from build123d import *

# Parameters (mm, degrees)
F1_DEPTH  = 10
F3_DEPTH  = 25.0000003725
F4_DEPTH  = 15
F5_R      = 13.75
F6_DEPTH  = 11.5
F7_DEPTH  = 7.5
F8_W      = 3
F8_H      = 12.169879545
F9_DEPTH  = 7
F10_W     = 3
F10_H     = 7.9815720619
F11_DEPTH = 4
F12_R     = 5
F13_R     = 5


# Not quite as in the source:
# - a feature names something its author has since deleted; it is built from what else it names


with BuildPart() as f1:
    # F0 (on Top) → F1 (new body)
    with BuildSketch(Plane.XY):
        with BuildLine():
            ThreePointArc((50, 15), (39.7487373415, 39.7487373415), (15, 50))
            Line((15, 50), (-15, 50))
            ThreePointArc((-15, 50), (-39.7487373415, 39.7487373415), (-50, 15))
            Line((-50, 15), (-50, -30))
            ThreePointArc((-50, -30), (-44.1421356237, -44.1421356237), (-30, -50))
            Line((-30, -50), (17.3621465266, -50))
            ThreePointArc((17.3621465266, -50), (19.1299134795, -49.267766953), (19.8621465266, -47.5))
            Line((19.8621465266, -47.5), (19.8621465266, -37.5))
            ThreePointArc((19.8621465266, -37.5), (19.1299134795, -35.732233047), (17.3621465266, -35))
            Line((17.3621465266, -35), (-30, -35))
            ThreePointArc((-30, -35), (-33.5355339059, -33.5355339059), (-35, -30))
            Line((-35, -30), (-35, 15))
            ThreePointArc((-35, 15), (-29.1421356237, 29.1421356237), (-15, 35))
            Line((-15, 35), (15, 35))
            ThreePointArc((15, 35), (29.1421356237, 29.1421356237), (35, 15))
            Line((35, 15), (35, -35))
            Line((35, -35), (35, -50))
            Line((35, -50), (50, -50))
            Line((50, -50), (50, 15))
        make_face()
    extrude(amount=F1_DEPTH)

    # F2 (on face) → F3 (cut)
    with BuildSketch(Plane.YZ.offset(50)):
        with BuildLine():
            ThreePointArc((-34.4148690401, 0), (-41.4859368519, 2.9289321881), (-44.4148690401, 10))
            Line((-44.4148690401, 10), (-50, 10))
            Line((-50, 10), (-50, 0))
            Line((-50, 0), (-34.4148690401, 0))
        make_face()
    extrude(amount=-F3_DEPTH, mode=Mode.SUBTRACT)

    # F2 (on face) → F4 (join)
    with BuildSketch(Plane.YZ.offset(50)):
        with BuildLine():
            Line((-10.5677563486, 86.0143546169), (-43.5051570601, 14.1673329256))
            ThreePointArc((-43.5051570601, 14.1673329256), (-44.1847943264, 12.1327353094), (-44.4148690401, 10))
            Line((-44.4148690401, 10), (-24.9867949218, 10))
            ThreePointArc((-24.9867949218, 10), (-29.1950209325, 12.299845589), (-29.5319389318, 17.0836664628))
            Line((-29.5319389318, 17.0836664628), (-0.1259929755, 81.2274541128))
            Line((-0.1259929755, 81.2274541128), (-10.5677563486, 86.0143546169))
        make_face()
    extrude(amount=-F4_DEPTH)

    # F5 (on face) → F6 (join)
    with BuildSketch(Plane(origin=(0, -41.3166681437, 18.9411282845), x_dir=(1, 0, 0), z_dir=(0, -0.909028802, 0.4167332926))):
        with BuildLine():
            ThreePointArc((-0.5725613731, 57.6122225326), (-5.3096309812, 69.0485202264), (-16.7459286749, 73.7855898345))
            ThreePointArc((-16.7459286749, 73.7855898345), (-32.9192959768, 57.6122225326), (-16.7459286749, 41.4388552308))
            ThreePointArc((-16.7459286749, 41.4388552308), (-5.3096309812, 46.1759248389), (-0.5725613731, 57.6122225326))
        make_face()
        with Locations((-16.7459286749, 57.6122225326)):
            Circle(F5_R, mode=Mode.SUBTRACT)
        with Locations((-16.7459286749, 57.6122225326)):
            Circle(F5_R)
        with BuildLine():
            Line((35, 41.4388552308), (35, 73.7855898345))
            Line((35, 73.7855898345), (-16.7459286749, 73.7855898345))
            ThreePointArc((-16.7459286749, 73.7855898345), (-5.3096309812, 69.0485202264), (-0.5725613731, 57.6122225326))
            ThreePointArc((-0.5725613731, 57.6122225326), (-5.3096309812, 46.1759248389), (-16.7459286749, 41.4388552308))
            Line((-16.7459286749, 41.4388552308), (35, 41.4388552308))
        make_face()
    extrude(amount=-F6_DEPTH)

    # F5 (on face) → F7 (cut)
    with BuildSketch(Plane(origin=(0, -41.3166681437, 18.9411282845), x_dir=(1, 0, 0), z_dir=(0, -0.909028802, 0.4167332926))):
        with Locations((-16.7459286749, 57.6122225326)):
            Circle(F5_R)
    extrude(amount=-F7_DEPTH, mode=Mode.SUBTRACT)

    # F8 (on face) → F9 (cut)
    with BuildSketch(Plane(origin=(0, -41.3166681437, 18.9411282845), x_dir=(1, 0, 0), z_dir=(0, -0.909028802, 0.4167332926))):
        with BuildLine():
            Line((2.0040713251, 56.1122225326), (2.0040713251, 59.1122225326))
            Line((2.0040713251, 59.1122225326), (2.0040713251, 61.1122225326))
            Line((2.0040713251, 61.1122225326), (-3.448842528, 61.1122225326))
            ThreePointArc((-3.448842528, 61.1122225326), (-3.109627224, 59.376813913), (-2.9959286749, 57.6122225326))
            ThreePointArc((-2.9959286749, 57.6122225326), (-3.109627224, 55.8476311523), (-3.448842528, 54.1122225326))
            Line((-3.448842528, 54.1122225326), (2.0040713251, 54.1122225326))
            Line((2.0040713251, 54.1122225326), (2.0040713251, 56.1122225326))
        make_face()
        with BuildLine():
            Line((36, 59.1122225326), (2.0040713251, 59.1122225326))
            Line((2.0040713251, 59.1122225326), (2.0040713251, 56.1122225326))
            Line((2.0040713251, 56.1122225326), (36, 56.1122225326))
            ThreePointArc((36, 56.1122225326), (39.5355339059, 54.6477564386), (41, 51.1122225326))
            Line((41, 51.1122225326), (41, -5.251533668))
            Line((41, -5.251533668), (44, -5.251533668))
            Line((44, -5.251533668), (44, 51.1122225326))
            ThreePointArc((44, 51.1122225326), (41.6568542495, 56.7690767821), (36, 59.1122225326))
        make_face()
        with Locations((42.5, -11.3364734405)):
            Rectangle(F8_W, F8_H)
    extrude(amount=-F9_DEPTH, mode=Mode.SUBTRACT)

    # F10 (on face) → F11 (cut)
    with BuildSketch(Plane(origin=(0, 0, 0), x_dir=(1, 0, 0), z_dir=(0, 0, -1))):
        with Locations((42.5, 38.4056550711)):
            Rectangle(F10_W, F10_H)
        with BuildLine():
            Line((44, 34.4148690401), (41, 34.4148690401))
            Line((41, 34.4148690401), (41, -38.4307490277))
            ThreePointArc((41, -38.4307490277), (42.5667640895, -36.5655632349), (44, -34.5959179423))
            Line((44, -34.5959179423), (44, 34.4148690401))
        make_face()
    extrude(amount=-F11_DEPTH, mode=Mode.SUBTRACT)

    # F12
    f12_edges = [f1.edges().sort_by_distance(p)[0] for p in [
        (42.5, -40.465722, 4),
    ]]
    fillet(f12_edges, radius=F12_R)

    # F13
    f13_edges = [f1.edges().sort_by_distance(p)[0] for p in [
        (50, -5.346875, 83.620904),
    ]]
    fillet(f13_edges, radius=F13_R)


solid = f1.part
Verification items for the finished model (mm, model axes). A direction names the side the tool comes from. Give positions to 0.01 mm unless a question says otherwise; leave off trailing zeros. Loops run counter-clockwise (first coordinate to the right, second up) from the corner with the lowest first, then second, coordinate; pieces in that order, holes last.
1) Depth check by flat-ended pin: pin 1 Ø0.9 at (x, y) = (42.5, -7.5) entering from -Z; pin 2 Ø10 at (y, z) = (-22, 41) entering from -X; pin 3 Ø2.5 at (y, z) = (-15, 66.5) entering from -X; pin 4 Ø5 at (x, y) = (37.5, 25) entering from -Z. Enter the tip coordinate at first touch or a pass-through.
2) Thickness scan on line 1 along X through (y, z) = (-41.5, 12.5); line 2 along Z through (x, y) = (39.5, 24); line 3 along Z through (x, y) = (43, -28). Record the ranges inside material, lowest first.
3) Draft check along Y on faces 6 (the flat face through (-16.94, -10.41, 68.36)), 7 (the flat face through (0, 50, 5)), 8 (the cylindrical face through (42.52, -36.84, 6.24)). Enter one of: pulls with the +Y half, pulls with the -Y half, needs draft (parallel to the pull), parting line crosses it, or undercut.
4) Sectioned sample at D-D, the plane z = 33. Enter the section's corners in (x, y).
5) Sectioned sample at B-B, the plane y = 5. Enter the section's corners in (x, z), then the cut area to 3 significant figures.
6) Set-up check for faces 1 (the flat face through (-0.684, -12.712, 73.056)), 2 (the flat face through (42, 2, 4)), 3 (the flat face through (-0.761, -15.629, 66.693)), 4 (the cylindrical face through (-33, -34, 5)), 5 (the flat face through (-35.5, 0.7, 0)): record each of +Z, -Z, +X, -X, +Y, -Y from which the full face is reachable in a straight line by a thin tool's end or side.
7) Sectioned sample at A-A, the plane x = 5.5. Enter the section's corners in (y, z), then the cut area to 3 significant figures.
8) Sectioned sample at C-C, the plane x = 25. Enter the section's corners in (y, z).
Answers:
1. pin 1: stops at z = 4
1. pin 2: stops at x = 35
1. pin 3: stops at x = -32.77
1. pin 4: stops at z = 0
2. line 1: x = 35 to 41, 44 to 50
2. line 2: z = 0 to 10
2. line 3: z = 4 to 11.01, 20.43 to 31.19
3. face 6: undercut
3. face 7: pulls with the +Y half
3. face 8: pulls with the -Y half
4. outline: (35, -34.87) - (41, -34.87) - (41, -27.17) - (44, -27.17) - (44, -34.87) - (50, -34.87) - (50, -22.24) - (35, -22.24) - close
5. outline: (-50, 0) - (-35, 0) - (-35, 10) - (-50, 10) - close; (35, 0) - (41, 0) - (41, 4) - (44, 4) - (44, 0) - (50, 0) - (50, 10) - (35, 10) - close
5. area: 288 mm2
6. face 1: -Y
6. face 2: -Z, +Y, -Y
6. face 3: none
6. face 4: +Z, -Z
6. face 5: -Z, +X, -X, +Y, -Y
7. outline: (-50, 0) - (-35, 0) - (-35, 10) - (-50, 10) - close; (-24.05, 56.61) - (-13.59, 51.82) - (-0.11, 81.22) - (-10.57, 86.01) - (-16.68, 72.68) - (-10.32, 69.76) - (-11.57, 67.03) - (-17.93, 69.95) - close; (35, 0) - (50, 0) - (50, 10) - (35, 10) - close
7. area: 651 mm2
8. outline: (-24.05, 56.61) - (-13.59, 51.82) - (-0.11, 81.22) - (-10.57, 86.01) - (-16.68, 72.68) - (-10.32, 69.76) - (-11.57, 67.03) - (-17.93, 69.95) - close; (32.32, 0) - (48.54, 0) - (48.54, 10) - (32.32, 10) - close
